from build123d import *

# Parameters (mm, degrees)
F1_DEPTH = 2.54
F2_DEPTH = 215.9


with BuildPart() as f1:
    # F0 (on Front) → F1 (new body)
    with BuildSketch(Plane.XZ):
        Polygon((-65.288178, -24.951821), (-65.288178, -126.551821), (-60.989264, -126.551821), (1232.651822, -126.551821), (1232.651822, 25.848179), (1232.651822, 127.448179), (-65.288178, 127.448179), align=None)
    extrude(amount=F1_DEPTH)

    # F0 (on Front) → F2 (join)
    with BuildSketch(Plane.XZ):
        Polygon((1235.191822, 129.988179), (-67.828178, 129.988179), (-67.828178, -24.951821), (-67.828178, -126.571611), (-65.288178, -126.551821), (-65.288178, -24.951821), (-65.288178, 127.448179), (1232.651822, 127.448179), (1232.651822, 25.848179), (1232.651822, -126.551821), (1235.191822, -126.551821), (1235.191822, -24.951821), align=None)
    extrude(amount=F2_DEPTH)


solid = f1.part
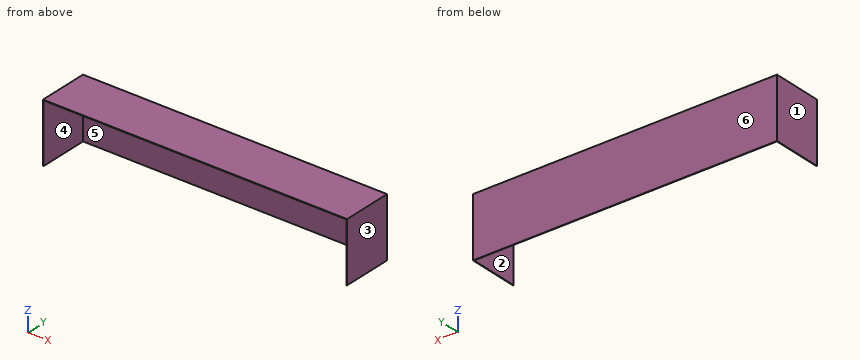
The model under review builds one solid part; all positions refer to its coordinate system, in mm. Face numbers are marked on the shaded views. A direction names the side the tool comes from. Give positions to 0.01 mm unless a question says otherwise; leave off trailing zeros. Order: outer loops, then holes, each group sorted by start corner. A loop starts at its lowest first (then second) coordinate and runs counter-clockwise, first axis right, second up. Notation, with made-up numbers: M 46.25,54 L 78.25,54 A14 ccw 78.25,72 Z; hole C 54.25,-14.75 d4. An arc over 180 degrees is marked long. Use one line per item in the form item = value. Start each with the question number.
Item 1: We need section B-B on y = -31.5. Give the boundary of the cut face in (x, z).
Item 2: We need section A-A on z = 59.5. Give the boundary of the cut face in (x, y).
Item 3: The part is to be moulded in two halves that separate along X. For the marked faces 1, 2, 3 and 4, say which applies: pulls with the +X half, pulls with the -X half, needs draft (parallel to the pull), parting line crosses it, or undercut.
Item 4: We need section C-C on x = 601.5. Give the boundary of the cut face in (y, z).
Item 5: For the marked faces 5 and 6, list the 3-axis set-ups (+Z, -Z, +X, -X, +Y, -Y) from which the entire face can be reached by the end or side of a thin tool; tool diameter is ignored.
Item 6: Insertion check: pin 1 Ø8 at (x, z) = (1099.5, -56.5) entering from +Y; pin 2 Ø4 at (x, y) = (984.5, -71.5) entering from -Z. Each pin has a flat end and moves straight along its axis. Give the tip position at first contact, or say it passes through.
Item 7: To check wall thickness, follow line 1 along X through (y, z) = (-181, 113); line 2 along Z through (x, y) = (105, -84); line 3 along Y through (x, z) = (1062, 104). State the ranges of each line that lie inside material, in increasing order. Write a range as from..to.
Completed:
q1.outline = M -67.83,-126.57 L -65.29,-126.55 L -65.29,127.45 L 1232.65,127.45 L 1232.65,-126.55 L 1235.19,-126.55 L 1235.19,129.99 L -67.83,129.99 Z
q2.outline = M -67.83,-215.9 L -65.29,-215.9 L -65.29,-2.54 L 1232.65,-2.54 L 1232.65,-215.9 L 1235.19,-215.9 L 1235.19,0 L -67.83,0 Z
q3.face_1 = pulls with the -X half
q3.face_2 = undercut
q3.face_3 = pulls with the +X half
q3.face_4 = undercut
q4.outline = M -215.9,127.45 L -2.54,127.45 L -2.54,-126.55 L 0,-126.55 L 0,129.99 L -215.9,129.99 Z
q5.face_5 = -Z, -Y
q5.face_6 = +Z, -Z, +X, -X, +Y
q6.pin_1 = 0
q6.pin_2 = 127.45
q7.line_1 = -67.83..-65.29, 1232.65..1235.19
q7.line_2 = 127.45..129.99
q7.line_3 = -2.54..0
